```python
from build123d import *

# Parameters (mm, degrees)
BOSS_EXTRUDE1_DEPTH = 40
SKETCH2_W           = 24.6
SKETCH2_H           = 9
CUT_EXTRUDE1_DEPTH  = 36
SKETCH3_R           = 3
CUT_EXTRUDE2_DEPTH  = 4.5


with BuildPart() as part:
    # Sketch1 → Boss-Extrude1 (new body)
    with BuildSketch(Plane.XY):
        with BuildLine():
            Line((-12, -7), (12, -7))
            ThreePointArc((12, -7), (14.121320344, -6.121320344), (15, -4))
            Line((15, -4), (15, 4))
            ThreePointArc((15, 4), (14.121320344, 6.121320344), (12, 7))
            Line((12, 7), (-12, 7))
            ThreePointArc((-12, 7), (-14.121320344, 6.121320344), (-15, 4))
            Line((-15, 4), (-15, -4))
            ThreePointArc((-15, -4), (-14.121320344, -6.121320344), (-12, -7))
        make_face()
    extrude(amount=BOSS_EXTRUDE1_DEPTH)

    # Sketch2 → Cut-Extrude1 (cut)
    with BuildSketch(Plane(origin=(0, 0, 0), x_dir=(-1, 0, 0), z_dir=(0, 0, -1))):
        Rectangle(SKETCH2_W, SKETCH2_H)
    extrude(amount=-CUT_EXTRUDE1_DEPTH, mode=Mode.SUBTRACT)

    # Sketch3 → Cut-Extrude2 (cut)
    with BuildSketch(Plane.XY.offset(40)):
        Circle(SKETCH3_R)
    extrude(amount=-CUT_EXTRUDE2_DEPTH, mode=Mode.SUBTRACT)


solid = part.part
```
Here's how the part is built. I have some questions about the finished solid (model axes, mm). A direction names the side the tool comes from. Coordinates: 2 decimals unless noted, no trailing zeros. Loops run counter-clockwise (first coordinate to the right, second up) from the corner with the lowest first, then second, coordinate; pieces in that order, holes last. Notation, with made-up numbers: (0.5, 56.5) - (17.5, 56.5) arc R21 cw to (17.5, 78.5) - close; hole circle Ø6 at (-18, 19). An arc over 180 degrees is marked (long way). Return JSON: item names as keys, results as strings. Group by question number.
Item 1: If we section it at C-C on z = 3: Write out the boundary of the cut face in (x, y), and give its area (3 significant figures).
Item 2: If we section it at A-A on y = 0: Write out the boundary of the cut face in (x, z), and give its area (3 significant figures).
Item 3: On a 3-axis mill with a long thin cutter (end or side, diameter ignored), from which of +Z, -Z, +X, -X, +Y, -Y can I reach the whole of each face in a straight line? I mean faces 5 (the face through (0, -7, 20)), 6 (the face through (12.3, 0, 18)). Say none if no direction works.
Item 4: If we section it at D-D on y = -3.5: Write out the boundary of the cut face in (x, z), and give its area (3 significant figures).
Item 5: If we section it at B-B on x = 0: Write out the boundary of the cut face in (y, z).
Item 6: Will these pins go through, and if not, where does the flat tip stop? P1, Ø2.5, axis at x = 5.5, y = -1.5, coming from the -Z side; P2, Ø5.5, axis at x = 0, y = 0, coming from the +Z side.
Item 7: I need wall thicknesses on line 1 (X direction, y = -2.5, z = 6); line 2 (Y direction, x = -4.5, z = 11.5); line 3 (Y direction, x = 0, z = 39.2). Which ranges of each line are inside material? Lowest first, please. Write a range as from..to.
Item 8: We'd pull the mould along X, two halves only. Please class faces 1 (the face through (14.1, -6.14, 19.72)), 2 (the face through (-3, 0, 38)), 3 (the face through (-15, 0, 20)), 4 (the face through (-12.3, 0, 18)): +X half, -X half, draft (parallel to the pull), parting line (faces both ways), or undercut.
Calculated:
{
 "1": {"outline": "(-15, -4) arc R3 ccw to (-12, -7) - (12, -7) arc R3 ccw to (15, -4) - (15, 4) arc R3 ccw to (12, 7) - (-12, 7) arc R3 ccw to (-15, 4) - close; hole (-12.3, -4.5) - (12.3, -4.5) - (12.3, 4.5) - (-12.3, 4.5) - close", "area": "191 mm^2"},
 "2": {"outline": "(-15, 0) - (-12.3, 0) - (-12.3, 36) - (-3, 36) - (-3, 40) - (-15, 40) - close; (3, 36) - (12.3, 36) - (12.3, 0) - (15, 0) - (15, 40) - (3, 40) - close", "area": "290 mm^2"},
 "3": {"face 5": "+Z, -Z, +X, -X, -Y", "face 6": "-Z"},
 "4": {"outline": "(-15, 0) - (-12.3, 0) - (-12.3, 36) - (12.3, 36) - (12.3, 0) - (15, 0) - (15, 40) - (-15, 40) - close", "area": "314 mm^2"},
 "5": {"outline": "(-7, 0) - (-4.5, 0) - (-4.5, 36) - (-3, 36) - (-3, 40) - (-7, 40) - close; (3, 36) - (4.5, 36) - (4.5, 0) - (7, 0) - (7, 40) - (3, 40) - close"},
 "6": {"P1": "stops at z = 36", "P2": "passes through"},
 "7": {"line 1": "x = -15..-12.3, 12.3..15", "line 2": "y = -7..-4.5, 4.5..7", "line 3": "y = -7..-3, 3..7"},
 "8": {"face 1": "+X half", "face 2": "undercut", "face 3": "-X half", "face 4": "undercut"}
}
